```python
from build123d import *

# Parameters (mm, degrees)
BOSS_EXTRUDE3_DEPTH = 1
BOSS_EXTRUDE4_DEPTH = 2
FILLET1_R           = 0.5


with BuildPart() as part:
    # Sketch1 → Boss-Extrude3 (new body)
    with BuildSketch(Plane.XY):
        Polygon((-0.414213562, 7), (5.585786438, 1), (-0.414213562, 1), (-11, 1), (-11, 7), align=None)
    extrude(amount=BOSS_EXTRUDE3_DEPTH)

    # Sketch4 → Boss-Extrude4 (add)
    with BuildSketch(Plane.XY.offset(1)):
        Polygon((-0.621320344, 6.5), (4.378679656, 1.5), (-0.621320344, 1.5), (-10.5, 1.5), (-10.5, 6.5), align=None)
    extrude(amount=BOSS_EXTRUDE4_DEPTH)

    # Fillet1
    fillet1_edges = [part.edges().sort_by_distance(p)[0] for p in [
        (-10.5, 6.5, 2),
        (-10.5, 1.5, 2),
        (4.378679656, 1.5, 2),
        (-0.621320344, 6.5, 2),
        (-10.5, 4, 3),
        (-3.060660172, 1.5, 3),
        (1.878679656, 4, 3),
        (-5.560660172, 6.5, 3),
    ]]
    fillet(fillet1_edges, radius=FILLET1_R)


solid = part.part
```
Check sheet for the modelled part. Datum: model origin and axes. Units: mm. A direction names the side the tool comes from. Coordinates: 2 decimals unless noted, no trailing zeros. Order: outer loops, then holes, each group sorted by start corner. A loop starts at its lowest first (then second) coordinate and runs counter-clockwise, first axis right, second up. Notation, with made-up numbers: (6.5, 38) -> (28.5, 38) arc R23 cw to (28.5, 52) -> close; hole circle Ø4 at (80.5, 74.25). An arc over 180 degrees is marked (long way). Write item = value, one per line. Start each with the question number.
1) Access from +Z, -Z, +X, -X, +Y, -Y to the whole of each face (thin tool, end or side, straight path). Record for faces 1 (the flat face through (1.5, 4.38, 1.74)), 2 (the flat face through (-3.9, 1.3, 1)), 3 (the flat face through (-5, 6.5, 2)).
2) Material ranges on L1, parallel to Y at x = -7.75, z = 1.95; L2, parallel to Z at x = -8.5, y = 6.55; L3, parallel to X at y = 3.6, z = 0.6, recorded low to high.
3) Go/stop test with flat-tipped pins: P1, Ø1.6, axis at x = -2, z = 2, coming from the -Y side; P2, Ø1.5, axis at x = -7, z = 2.5, coming from the +Y side; P3, Ø1.5, axis at x = 3.5, y = 5, coming from the +Z side. Record where each tip stops, or that it passes through.
4) Cross-section at C-C (y = 1.7). Enter the section's corners in (x, z).
5) Cross-section at D-D (z = 2.65). Enter the section's corners in (x, y), then the cut area to 3 significant figures.
6) Cross-section at A-A (z = 1.35). Enter the section's corners in (x, y), then the cut area to 3 significant figures.
7) Cross-section at B-B (x = -1). Enter the section's corners in (y, z).
Ans:
q1.face_1 = +Z, +X, +Y
q1.face_2 = +Z
q1.face_3 = +Z, +X, -X, +Y
q2.L1 = 1.5 to 6.5
q2.L2 = 0 to 1
q2.L3 = -11 to 2.99
q3.P1 = 1.5
q3.P2 = 6.5
q3.P3 = through
q4.outline = (-11, 0) -> (4.89, 0) -> (4.89, 1) -> (3.57, 1) -> (3.57, 2.5) arc R0.4 ccw to (3.17, 2.9) -> (-10, 2.9) arc R0.4 ccw to (-10.4, 2.5) -> (-10.4, 1) -> (-11, 1) -> close
q5.outline = (-10.48, 2) arc R0.48 ccw to (-10, 1.52) -> (3.17, 1.52) arc R0.48 ccw to (3.51, 2.34) -> (-0.49, 6.34) arc R0.48 ccw to (-0.83, 6.48) -> (-10, 6.48) arc R0.48 ccw to (-10.48, 6) -> close
q5.area = 60.7 mm²
q6.outline = (-10.5, 2) arc R0.5 ccw to (-10, 1.5) -> (3.17, 1.5) arc R0.5 ccw to (3.53, 2.35) -> (-0.47, 6.35) arc R0.5 ccw to (-0.83, 6.5) -> (-10, 6.5) arc R0.5 ccw to (-10.5, 6) -> close
q6.area = 61.5 mm²
q7.outline = (1, 0) -> (7, 0) -> (7, 1) -> (6.5, 1) -> (6.5, 2.5) arc R0.5 ccw to (6, 3) -> (2, 3) arc R0.5 ccw to (1.5, 2.5) -> (1.5, 1) -> (1, 1) -> close
